CAD build for the part. Positions are in the model's coordinates, mm. Face numbers are marked on the shaded views. A direction names the side the tool comes from. Give positions to 0.01 mm unless a question says otherwise; leave off trailing zeros. Order: outer loops, then holes, each group sorted by start corner. A loop starts at its lowest first (then second) coordinate and runs counter-clockwise, first axis right, second up. Notation, with made-up numbers: (83.25, -2) -> (98.25, -2) arc R23 cw to (98.25, 17) -> close; hole circle Ø2 at (65.5, 26). An arc over 180 degrees is marked (long way). Use one line per item in the form item = value. Start each with the question number.
1) Cut at B-B, the plane x = 293.5. Give the cut face in (y, z).
2) Probe line 1 (Z direction, x = 292.5, y = -148.5); line 2 (X direction, y = -154, z = -2); line 3 (Z direction, x = 274.5, y = -143.5). List the from-to ranges inside material, lowest first.
3) Mould opens along Z. For the marked faces 1, 2, 3 and 4 say: pulls with the +Z half, pulls with the -Z half, needs draft (parallel to the pull), parting line crosses it, or undercut.
4) Tool access for the marked faces 5 and 6: list every direction of +Z, -Z, +X, -X, +Y, -Y with a clear straight run to the whole face (end or side of a thin tool).
5) Cut at D-D, the plane y = -153. Give the cut face in (x, z), and give its area (3 significant figures).
6) Cut at C-C, the plane z = -12. Give the cut face in (x, y), and give its area (3 significant figures).
7) Drop flat-ended pins along their axis: P1, Ø4, axis at x = 294, y = -146, coming from the +Z side; P2, Ø1.3, axis at y = -151.47, z = 2.9, coming from the -X side; P3, Ø4, axis at y = -148.57, z = -12, coming from the +X side; P4, Ø1.5, axis at x = 280.5, z = 6, coming from the -Y side. Give the stop position or say it passes through.
8) Cut at A-A, the plane z = 0. Give the cut face in (x, y), and give its area (3 significant figures).
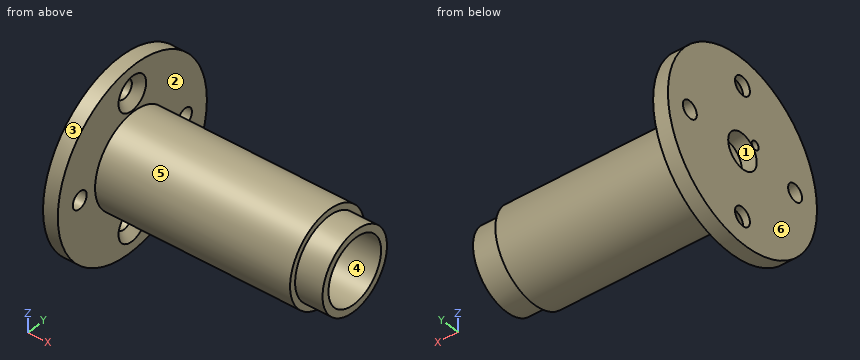
from build123d import *

# Parameters (mm, degrees)
CUT_EXTRUDE1_REACH                                  = 4.7
SKETCH4_R                                           = 1.5875
CSK_FOR_M3_COUNTERSUNK_FLAT_HEAD_SCREW1_D           = 3.4
CSK_FOR_M3_COUNTERSUNK_FLAT_HEAD_SCREW1_DEPTH       = 10
CSK_FOR_M3_COUNTERSUNK_FLAT_HEAD_SCREW1_CSINK_D     = 6.3
CSK_FOR_M3_COUNTERSUNK_FLAT_HEAD_SCREW1_CSINK_ANGLE = 90
CSK_FOR_M3_COUNTERSUNK_FLAT_HEAD_SCREW1_TIP         = 1.021463052
SKETCH14_R                                          = 0.8
CUT_EXTRUDE3_DEPTH                                  = 10


with BuildPart() as part:
    # Sketch3 → Revolve19 (revolve)
    with BuildSketch(Plane.XY):
        Polygon((299.808388758, -140.073704322), (264.258388758, -140.073704322), (264.258388758, -131.573704322), (261.558388758, -131.573704322), (261.558388758, -143.823704322), (261.558388758, -145.323704322), (262.558388758, -145.323704322), (264.258388758, -145.323704322), (264.258388758, -142.573704322), (304.808388758, -142.573704322), (304.808388758, -141.223704322), (299.808388758, -141.223704322), align=None)
    revolve(axis=Axis((227.370475166, -148.573704322, 0), (1, 0, 0)))

    # Sketch4 → Cut-Extrude1 (cut, up to next)
    with BuildSketch(Plane(origin=(264.258388758, 0, 0), x_dir=(0, 0, -1), z_dir=(1, 0, 0)), mode=Mode.PRIVATE) as cut_extrude1_sk1:
        with Locations((0, -136.573704322)):
            Circle(SKETCH4_R)
    cut_extrude1_tool1 = extrude(cut_extrude1_sk1.sketch, amount=-CUT_EXTRUDE1_REACH, mode=Mode.PRIVATE) & part.part
    add(cut_extrude1_tool1.solids().sort_by_distance((264.258389, -136.573704, 0))[0], mode=Mode.SUBTRACT)
    # Sketch4 → Cut-Extrude1 (cut, up to next)
    with BuildSketch(Plane(origin=(264.258388758, 0, 0), x_dir=(0, 0, -1), z_dir=(1, 0, 0)), mode=Mode.PRIVATE) as cut_extrude1_sk2:
        with Locations((0, -160.573704322)):
            Circle(SKETCH4_R)
    cut_extrude1_tool2 = extrude(cut_extrude1_sk2.sketch, amount=-CUT_EXTRUDE1_REACH, mode=Mode.PRIVATE) & part.part
    add(cut_extrude1_tool2.solids().sort_by_distance((264.258389, -160.573704, 0))[0], mode=Mode.SUBTRACT)

    # CSK for M3 Countersunk Flat Head Screw1
    with Locations(Plane(origin=(264.258388758, 0, 0), x_dir=(0, 0, -1), z_dir=(1, 0, 0))):
        with Locations((-12, -148.573704322), (12, -148.573704322)):
            CounterSinkHole(CSK_FOR_M3_COUNTERSUNK_FLAT_HEAD_SCREW1_D / 2, CSK_FOR_M3_COUNTERSUNK_FLAT_HEAD_SCREW1_CSINK_D / 2, depth=CSK_FOR_M3_COUNTERSUNK_FLAT_HEAD_SCREW1_DEPTH, counter_sink_angle=CSK_FOR_M3_COUNTERSUNK_FLAT_HEAD_SCREW1_CSINK_ANGLE)
            with Locations((0, 0, -(CSK_FOR_M3_COUNTERSUNK_FLAT_HEAD_SCREW1_DEPTH + CSK_FOR_M3_COUNTERSUNK_FLAT_HEAD_SCREW1_TIP / 2))):  # 118° drill point
                Cone(0, CSK_FOR_M3_COUNTERSUNK_FLAT_HEAD_SCREW1_D / 2, CSK_FOR_M3_COUNTERSUNK_FLAT_HEAD_SCREW1_TIP, mode=Mode.SUBTRACT)

    # Sketch14 → Cut-Extrude3 (cut)
    with BuildSketch(Plane(origin=(264.258388758, 0, 0), x_dir=(0, 0, -1), z_dir=(1, 0, 0))):
        with Locations((-2.899137803, -151.472842125)):
            Circle(SKETCH14_R)
    extrude(amount=-CUT_EXTRUDE3_DEPTH, mode=Mode.SUBTRACT)


solid = part.part
Result:
q1.outline = circle Ø17 at (-148.57, 0); hole circle Ø12 at (-148.57, 0)
q2.line_1 = -8.5 to -6, 6 to 8.5
q2.line_2 = 261.56 to 264.26
q2.line_3 = -6.82 to -3.2, 3.2 to 6.82
q3.face_1 = undercut
q3.face_2 = needs draft
q3.face_3 = parting line crosses it
q3.face_4 = undercut
q4.face_5 = +X
q4.face_6 = +Z, -Z, -X, +Y, -Y
q5.outline = (261.56, -16.41) -> (264.26, -16.41) -> (264.26, -7.26) -> (299.81, -7.26) -> (299.81, -5.87) -> (304.81, -5.87) -> (304.81, -4.05) -> (264.26, -4.05) -> (264.26, 4.05) -> (304.81, 4.05) -> (304.81, 5.87) -> (299.81, 5.87) -> (299.81, 7.26) -> (264.26, 7.26) -> (264.26, 16.41) -> (261.56, 16.41) -> close
q5.area = 335 mm²
q6.outline = (261.56, -160.62) -> (264.26, -160.62) -> (264.26, -151.72) -> (262.81, -150.27) -> (261.56, -150.27) -> close; (261.56, -146.87) -> (262.81, -146.87) -> (264.26, -145.42) -> (264.26, -136.53) -> (261.56, -136.53) -> close
q6.area = 53.7 mm²
q7.P1 = 8.48
q7.P2 = through
q7.P3 = 263.11
q7.P4 = -155.26
q8.outline = (261.56, -165.57) -> (264.26, -165.57) -> (264.26, -162.16) -> (261.56, -162.16) -> close; (261.56, -158.99) -> (264.26, -158.99) -> (264.26, -157.07) -> (299.81, -157.07) -> (299.81, -155.92) -> (304.81, -155.92) -> (304.81, -154.57) -> (264.26, -154.57) -> (264.26, -151.82) -> (261.56, -151.82) -> close; (261.56, -145.32) -> (264.26, -145.32) -> (264.26, -142.57) -> (304.81, -142.57) -> (304.81, -141.22) -> (299.81, -141.22) -> (299.81, -140.07) -> (264.26, -140.07) -> (264.26, -138.16) -> (261.56, -138.16) -> close; (261.56, -134.99) -> (264.26, -134.99) -> (264.26, -131.57) -> (261.56, -131.57) -> close
q8.area = 248 mm²
